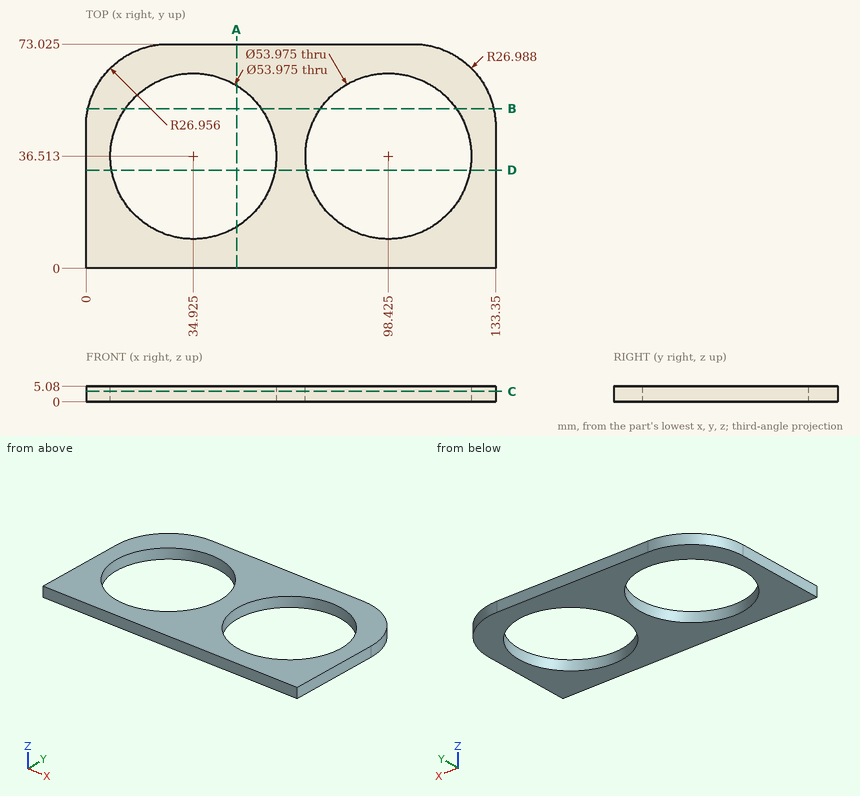
Source: three-view drawing plus pictorial views. Frame: mm from the lowest corner of the part. Give positions to 0.01 mm unless a question says otherwise; leave off trailing zeros. Order: outer loops, then holes, each group sorted by start corner. A loop starts at its lowest first (then second) coordinate and runs counter-clockwise, first axis right, second up. Notation, with made-up numbers: (35.25, -35.5) -> (91.25, -35.5) arc R19 ccw to (91.25, -18.5) -> close; hole circle Ø9 at (27.5, 49.5). An arc over 180 degrees is marked (long way). Put each result on its own line as item: value.
Q1. Section D-D, the plane y = 32. Return loops of the section in (x, z).
Here are the results:
outline: (0, 0) -> (8.32, 0) -> (8.32, 5.08) -> (0, 5.08) -> close; (61.53, 0) -> (71.82, 0) -> (71.82, 5.08) -> (61.53, 5.08) -> close; (125.03, 0) -> (133.35, 0) -> (133.35, 5.08) -> (125.03, 5.08) -> close
Q2. Material intervals for L1, parallel to X at y = 37, z = 2.25; L2, parallel to X at y = 31, z = 3.9; L3, parallel to Y at x = 33.5, z = 1.4 (1 decimal), sorted ascending.
Here are the results:
L1: x = 0 to 7.94, 61.91 to 71.44, 125.41 to 133.35
L2: x = 0 to 8.51, 61.34 to 72.01, 124.84 to 133.35
L3: y = 0 to 9.6, 63.5 to 73
Q3. Section C-C, the plane z = 3.45. Count the separate pieces of the cut face and the enclosed holes in it, then the cut area to 3 significant figures.
Here are the results:
separate pieces: 1
enclosed holes: 2
area: 4,850 mm^2
Q4. Pin query (flat end, axial travel): pin 1 (10 mm diameter, centred on x = 118.5, y = 23.5, fed in from -Z). Return the tip coordinate at first contact, or that it passes through.
Here are the results:
pin 1: stops at z = 0
Q5. Section B-B, the plane y = 52. Return loops of the section in (x, z).
Here are the results:
outline: (0.66, 0) -> (12.82, 0) -> (12.82, 5.08) -> (0.66, 5.08) -> close; (57.03, 0) -> (76.32, 0) -> (76.32, 5.08) -> (57.03, 5.08) -> close; (120.53, 0) -> (132.68, 0) -> (132.68, 5.08) -> (120.53, 5.08) -> close
Q6. Section A-A, the plane x = 49. Return loops of the section in (y, z) (1 decimal).
Here are the results:
outline: (0, 0) -> (13.5, 0) -> (13.5, 5.1) -> (0, 5.1) -> close; (59.5, 0) -> (73, 0) -> (73, 5.1) -> (59.5, 5.1) -> close
